The listing builds one solid part. Answer for the finished solid, in the listing's coordinates (mm). A direction names the side the tool comes from. Coordinates: 2 decimals unless noted, no trailing zeros. Order: outer loops, then holes, each group sorted by start corner. A loop starts at its lowest first (then second) coordinate and runs counter-clockwise, first axis right, second up. Notation, with made-up numbers: (45.25, 62.5) - (59.25, 62.5) arc R30 cw to (59.25, 85.5) - close; hole circle Ø1 at (-17.5, 24.25). An arc over 180 degrees is marked (long way). One line per item, written item: value. Start each with the question number.
```python
from build123d import *

# Parameters (mm, degrees)
ESQUISSE1_W             = 82
ESQUISSE1_H             = 49
BOSS_EXTRU_1_DEPTH      = 3
ESQUISSE2_W             = 38.309373872
ESQUISSE2_H             = 3
BOSS_EXTRU_2_DEPTH      = 48
ESQUISSE3_R             = 15.255971645
ENL_V_MAT_EXTRU_1_DEPTH = 96.571962416
ESQUISSE4_W             = 33.801324292
ESQUISSE4_H             = 8.092552901
ENL_V_MAT_EXTRU_2_DEPTH = 96.571962416
BOSS_EXTRU_3_DEPTH      = 5
BOSS_EXTRU_4_DEPTH      = 5
ESQUISSE8_R             = 1.2
ENL_V_MAT_EXTRU_3_DEPTH = 99.784235864
BOSS_EXTRU_6_START      = -38.309374
ESQUISSE9_W             = 5.724168344
ESQUISSE9_H             = 4
BOSS_EXTRU_6_DEPTH      = 38.309374
BOSS_EXTRU_7_DEPTH      = 4
ESQUISSE11_R            = 1.2
ENL_V_MAT_EXTRU_4_DEPTH = 99.784235864
ESQUISSE12_W            = 59.88479499
ESQUISSE12_H            = 26.036139414
ENL_V_MAT_EXTRU_5_DEPTH = 100.590767548


with BuildPart() as part:
    # Esquisse1 → Boss.-Extru.1 (new body)
    with BuildSketch(Plane.XY):
        with Locations((41, 24.5)):
            Rectangle(ESQUISSE1_W, ESQUISSE1_H)
    extrude(amount=BOSS_EXTRU_1_DEPTH)

    # Esquisse2 → Boss.-Extru.2 (add)
    with BuildSketch(Plane.XZ):
        with Locations((41, 1.5)):
            Rectangle(ESQUISSE2_W, ESQUISSE2_H)
    extrude(amount=BOSS_EXTRU_2_DEPTH)

    # Esquisse3 → Enlèv. mat.-Extru.1 (cut, through all)
    with BuildSketch(Plane(origin=(0, 0, 0), x_dir=(-1, 0, 0), z_dir=(0, 0, -1))):
        with Locations((-41.103242704, -23.088178639)):
            Circle(ESQUISSE3_R)
    extrude(amount=-ENL_V_MAT_EXTRU_1_DEPTH, mode=Mode.SUBTRACT)

    # Esquisse4 → Enlèv. mat.-Extru.2 (cut, through all)
    with BuildSketch(Plane(origin=(0, 0, 0), x_dir=(-1, 0, 0), z_dir=(0, 0, -1))):
        with Locations((-41, 44.953723549)):
            Rectangle(ESQUISSE4_W, ESQUISSE4_H)
    extrude(amount=-ENL_V_MAT_EXTRU_2_DEPTH, mode=Mode.SUBTRACT)

    # Esquisse5 → Boss.-Extru.3 (add)
    with BuildSketch(Plane(origin=(82, 0, 0), x_dir=(0, 0, -1), z_dir=(1, 0, 0))):
        Polygon((0, 49), (0, 24.5), (25.165954286, 36.75), align=None)
    extrude(amount=-BOSS_EXTRU_3_DEPTH)

    # Esquisse6 → Boss.-Extru.4 (add)
    with BuildSketch(Plane.ZY):
        Polygon((0, 49), (0, 24.5), (-25.165954286, 36.75), align=None)
    extrude(amount=-BOSS_EXTRU_4_DEPTH)

    # Esquisse8 → Enlèv. mat.-Extru.3 (cut, through all)
    with BuildSketch(Plane(origin=(0, 0, 0), x_dir=(-1, 0, 0), z_dir=(0, 0, -1))):
        with Locations((-41.11564979, -2.509917341)):
            Circle(ESQUISSE8_R)
    extrude(amount=-ENL_V_MAT_EXTRU_3_DEPTH, mode=Mode.SUBTRACT)

    # Esquisse9 → Boss.-Extru.6 (add)
    with BuildSketch(Plane.ZY.offset(-21.845313064).offset(BOSS_EXTRU_6_START)):
        with Locations((0.137915828, -39.687870455)):
            Rectangle(ESQUISSE9_W, ESQUISSE9_H)
    extrude(amount=BOSS_EXTRU_6_DEPTH)

    # Esquisse10 → Boss.-Extru.7 (add)
    with BuildSketch(Plane.XZ.offset(41.687870455)):
        Polygon((21.845313064, -2.724168344), (60.154686936, -2.724168344), (41, -25.159658009), align=None)
    extrude(amount=-BOSS_EXTRU_7_DEPTH)

    # Esquisse11 → Enlèv. mat.-Extru.4 (cut, through all)
    with BuildSketch(Plane(origin=(0, 0, 0), x_dir=(-1, 0, 0), z_dir=(0, 0, -1))):
        with Locations((-41, -44.843935227)):
            Circle(ESQUISSE11_R)
    extrude(amount=-ENL_V_MAT_EXTRU_4_DEPTH, mode=Mode.SUBTRACT)

    # Esquisse12 → Enlèv. mat.-Extru.5 (cut, through all)
    with BuildSketch(Plane.XY.offset(3)):
        with Locations((41.057824895, 19.798764879)):
            Rectangle(ESQUISSE12_W, ESQUISSE12_H)
    extrude(amount=-ENL_V_MAT_EXTRU_5_DEPTH, mode=Mode.SUBTRACT)


solid = part.part
```
(1) For a pull along Y with two mould halves and no side action, classify faces 5 (the face through (40, 6, 0)), 6 (the face through (71, 0, 1)), 7 (the face through (41, 32.817, 2)) as pulls with the +Y half, pulls with the -Y half, needs draft (parallel to the pull), parting line crosses it, or undercut.
(2) The part is cut by section D-D on y = -40. Determine the outline of the cut face in (x, z), plus the area to 3 significant figures.
(3) Flat-ended cylindrical pins translate along their axes: pin 1 Ø8 at (x, z) = (40, -5.5) entering from +Y; pin 2 Ø1 at (x, z) = (43, 0) entering from +Y; pin 3 Ø3.5 at (x, z) = (75, 1.5) entering from -Y. Find the tip coordinate at first contact, or state that the pin passes through.
(4) The part is cut by section B-B on y = 18. Determine the outline of the cut face in (x, z), plus the area to 3 significant figures.
(5) Consider probe 1 along Y at (x, z) = (41, 1.05); probe 2 along X at (y, z) = (42.5, -9.75); probe 3 along Y at (x, z) = (53, 2.25). Determine where each line is inside the solid, lowest interval first.
(6) The part is cut by section A-A on x = 15. Determine the outline of the cut face in (y, z).
(7) For faces 1 (the face through (42.314, -2.457, 1.479)), 2 (the face through (77, 37, -10)), 3 (the face through (57.901, 45, 1)), 4 (the face through (41, -41.688, -10)), determine the directions among +Z, -Z, +X, -X, +Y, -Y from which every point of the face is accessible in a straight line to the end or side of a thin tool.
(8) The part is cut by section C-C on z = -10.25. Determine the outline of the cut face in (x, y).
Completed:
1. face 5: needs draft
1. face 6: pulls with the -Y half
1. face 7: undercut
2. outline: (21.85, -2.72) - (41, -25.16) - (60.15, -2.72) - (60.15, 3) - (21.85, 3) - close
2. area: 649 mm2
3. pin 1: stops at y = -37.69
3. pin 2: stops at y = 40.91
3. pin 3: stops at y = 0
4. outline: (0, 0) - (11.12, 0) - (11.12, 3) - (0, 3) - close; (71, 0) - (82, 0) - (82, 3) - (71, 3) - close
4. area: 66.3 mm2
5. probe 1: y = -48 to -46.04, -43.64 to -37.69, -7.83 to -3.7, -1.32 to 6.78, 32.82 to 40.91
5. probe 2: x = 0 to 5, 77 to 82
5. probe 3: y = -48 to -32.64, -13.54 to 6.78, 32.82 to 40.91
6. outline: (0, 0) - (6.78, 0) - (6.78, 3) - (0, 3) - close; (32.82, 0) - (49, 0) - (49, 3) - (32.82, 3) - close
7. face 1: +Z, -Z
7. face 2: -Z, +Y, -Y
7. face 3: +Z, -Z, +Y
7. face 4: -Z, +X, -X, -Y
8. outline: (0, 29.49) - (5, 29.49) - (5, 44.01) - (0, 44.01) - close; (28.27, -41.69) - (53.73, -41.69) - (53.73, -37.69) - (28.27, -37.69) - close; (77, 29.49) - (82, 29.49) - (82, 44.01) - (77, 44.01) - close
